The listing builds one solid part. Answer for the finished solid, in the listing's coordinates (mm). Give positions to 0.01 mm unless a question says otherwise; leave off trailing zeros. Order: outer loops, then holes, each group sorted by start corner. A loop starts at its lowest first (then second) coordinate and runs counter-clockwise, first axis right, second up. Notation, with made-up numbers: M -15.75,-29.75 L 1.25,-29.75 A12 cw 1.25,-16.75 Z; hole C 19,47.25 d1. An arc over 180 degrees is marked long. Answer as a JSON object with one key per item and string values. Group by question number.
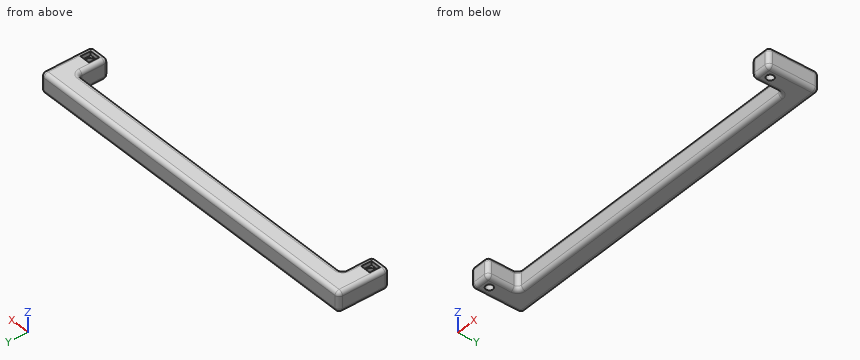
```python
from build123d import *

# Parameters (mm, degrees)
SKETCH1_W           = 224.4725
SKETCH1_H           = 12.7
BOSS_EXTRUDE1_DEPTH = 12.7
SKETCH2_W           = 12.7
SKETCH2_H           = 12.7
BOSS_EXTRUDE2_DEPTH = 19.05
SKETCH3_R           = 2.286
CUT_EXTRUDE1_DEPTH  = 226.63708861
SKETCH4_W           = 6.35
SKETCH4_H           = 6.35
CUT_EXTRUDE2_DEPTH  = 2.54
FILLET1_R           = 2.54


with BuildPart() as part:
    # Sketch1 → Boss-Extrude1 (new body)
    with BuildSketch(Plane.XY):
        with Locations((112.23625, 6.35)):
            Rectangle(SKETCH1_W, SKETCH1_H)
    extrude(amount=BOSS_EXTRUDE1_DEPTH)

    # Sketch2 → Boss-Extrude2 (add)
    with BuildSketch(Plane.XZ):
        with Locations((6.35, 6.35)):
            Rectangle(SKETCH2_W, SKETCH2_H)
    boss_extrude2 = extrude(amount=BOSS_EXTRUDE2_DEPTH)

    # Sketch3 → Cut-Extrude1 (cut, through all)
    with BuildSketch(Plane.XY.offset(12.7)):
        with Locations((6.35, -12.7)):
            Circle(SKETCH3_R)
    cut_extrude1 = extrude(amount=-CUT_EXTRUDE1_DEPTH, mode=Mode.SUBTRACT)

    # Sketch4 → Cut-Extrude2 (cut)
    with BuildSketch(Plane.XY.offset(12.7)):
        with Locations((6.35, -12.7)):
            Rectangle(SKETCH4_W, SKETCH4_H)
    cut_extrude2 = extrude(amount=-CUT_EXTRUDE2_DEPTH, mode=Mode.SUBTRACT)

    # Mirror1: Boss-Extrude2, Cut-Extrude1, Cut-Extrude2 across plane
    add(boss_extrude2.mirror(Plane.ZY.offset(-112.23625)))
    add(cut_extrude1.mirror(Plane.ZY.offset(-112.23625)), mode=Mode.SUBTRACT)
    add(cut_extrude2.mirror(Plane.ZY.offset(-112.23625)), mode=Mode.SUBTRACT)

    # Fillet1
    fillet1_edges = [part.edges().sort_by_distance(p)[0] for p in [
        (224.4725, -3.175, 12.7),
        (112.23625, 0, 0),
        (112.23625, 0, 12.7),
        (12.7, 0, 6.35),
        (112.23625, 12.7, 12.7),
        (12.7, -9.525, 0),
        (12.7, -9.525, 12.7),
        (0, -19.05, 6.35),
        (6.35, -19.05, 0),
        (12.7, -19.05, 6.35),
        (6.35, -19.05, 12.7),
        (0, -3.175, 12.7),
        (112.23625, 12.7, 0),
        (224.4725, -19.05, 6.35),
        (218.1225, -19.05, 12.7),
        (211.7725, -19.05, 6.35),
        (211.7725, -9.525, 12.7),
        (218.1225, -19.05, 0),
        (211.7725, -9.525, 0),
        (211.7725, 0, 6.35),
        (224.4725, -3.175, 0),
        (0, -3.175, 0),
        (0, 12.7, 6.35),
        (224.4725, 12.7, 6.35),
    ]]
    fillet(fillet1_edges, radius=FILLET1_R)


solid = part.part
```
Item 1: Section B-B (x = 6.35) is taken. Determine the outline of the cut face in (y, z) (3 decimals), and give its area (3 significant figures).
Item 2: Flat-ended cylindrical pins translate along their axes: P1, Ø1, axis at x = 143, z = 3, coming from the -Y side; P2, Ø3, axis at x = 217.5, y = -13.5, coming from the +Z side; P3, Ø2, axis at y = -9.5, z = 11, coming from the +X side; P4, Ø1.3, axis at y = -12, z = 11.5, coming from the +X side. Find the tip coordinate at first contact, or state that the pin passes through.
Item 3: Section D-D (x = 110) is taken. Determine the outline of the cut face in (y, z), and give its area (3 significant figures).
Item 4: Section C-C (z = 7.5) is taken. Determine the outline of the cut face in (x, y), and give its area (3 significant figures).
Item 5: Section A-A (y = -12.7) is taken. Count the separate pieces of the cut face and the enclosed holes in it, and give its area (3 significant figures).
Item 6: Consider probe 1 along Y at (x, z) = (6.35, 6.75); probe 2 along X at (y, z) = (-12, 3.5); probe 3 along X at (y, z) = (-13, 11.25) (1 decimal). Determine where each line is inside the solid, lowest interval first. Write a range as from..to.
Values found:
{
 "1": {"outline": "M -19.05,2.54 A2.54 ccw -16.51,0 L -14.986,0 L -14.986,10.16 L -15.875,10.16 L -15.875,12.7 L -16.51,12.7 A2.54 ccw -19.05,10.16 Z; M -10.414,0 L 10.16,0 A2.54 ccw 12.7,2.54 L 12.7,10.16 A2.54 ccw 10.16,12.7 L -9.525,12.7 L -9.525,10.16 L -10.414,10.16 Z", "area": "335 mm^2"},
 "2": {"P1": "stops at y = 0", "P2": "stops at z = 10.16", "P3": "stops at x = 224.47", "P4": "stops at x = 224.38"},
 "3": {"outline": "M 0,2.54 A2.54 ccw 2.54,0 L 10.16,0 A2.54 ccw 12.7,2.54 L 12.7,10.16 A2.54 ccw 10.16,12.7 L 2.54,12.7 A2.54 ccw 0,10.16 Z", "area": "156 mm^2"},
 "4": {"outline": "M 0,-16.51 A2.54 ccw 2.54,-19.05 L 10.16,-19.05 A2.54 ccw 12.7,-16.51 L 12.7,-2.54 A2.54 cw 15.24,0 L 209.23,0 A2.54 cw 211.77,-2.54 L 211.77,-16.51 A2.54 ccw 214.31,-19.05 L 221.93,-19.05 A2.54 ccw 224.47,-16.51 L 224.47,10.16 A2.54 ccw 221.93,12.7 L 2.54,12.7 A2.54 ccw 0,10.16 Z; hole C 6.35,-12.7 d4.57; hole C 218.12,-12.7 d4.57", "area": "3,300 mm^2"},
 "5": {"separate pieces": "4", "enclosed holes": "0", "area": "186 mm^2"},
 "6": {"probe 1": "y = -19.05..-14.99, -10.41..12.7", "probe 2": "x = 0..4.17, 8.53..12.7, 211.77..215.95, 220.3..224.47", "probe 3": "x = 0.2..3.2, 9.5..12.5, 212..214.9, 221.3..224.2"}
}
